Check sheet for the modelled part. Datum: model origin and axes. Units: mm. Face numbers are marked on the shaded views. A direction names the side the tool comes from. Round coordinates to 2 decimals unless told otherwise and drop trailing zeros. Order: outer loops, then holes, each group sorted by start corner. A loop starts at its lowest first (then second) coordinate and runs counter-clockwise, first axis right, second up. Notation, with made-up numbers: (67, 17) -> (115, 17) arc R13 ccw to (115, 38) -> close; hole circle Ø4 at (63.5, -8.75). An arc over 180 degrees is marked (long way). Answer in a Markdown table with one row per item. Add a question column.
1. Sectioned sample at D-D, the plane z = -20. Record the boundary of the cut face in (x, y), then the cut area to 3 significant figures.
2. Draft check along Z on the marked faces 1, 2, 3 and 4. Enter one of: +Z half, -Z half, draft (parallel to the pull), parting line (faces both ways), or undercut.
3. Material ranges on L1, parallel to Z at x = 0, y = 18; L2, parallel to X at y = -5.5, z = -19; L3, parallel to Y at x = -18.5, z = -28.5, recorded low to high. Write a range as from..to.
4. Sectioned sample at C-C, the plane y = 43. Record the boundary of the cut face in (x, z), then the cut area to 3 significant figures.
5. Sectioned sample at B-B, the plane z = -29. Record the boundary of the cut face in (x, y).
6. Sectioned sample at A-A, the plane x = 0. Record the boundary of the cut face in (y, z), then the cut area to 3 significant figures.
7. Access from +Z, -Z, +X, -X, +Y, -Y to the whole of each face (thin tool, end or side, straight path). Record for the marked faces 5, 6 and 7.
8. Depth check by flat-ended pin: P1, Ø4, axis at y = 41.5, z = 2.5, coming from the -X side; P2, Ø1, axis at y = 7.5, z = 3.5, coming from the -X side; P3, Ø1, axis at x = 11.5, y = 27.5, coming from the -Z side; P4, Ø8, axis at x = -8.5, z = -7, coming from the -Y side. Enter the tip coordinate at first touch or a pass-through.
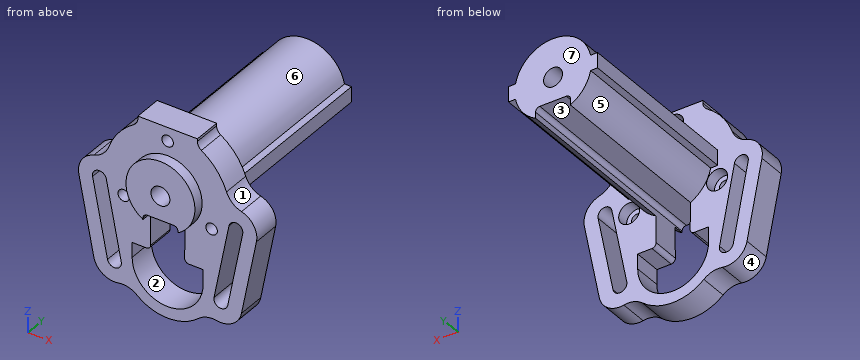
```python
from build123d import *

# Parameters (mm, degrees)
F1_DEPTH  = 8
F2_R      = 9.85
F3_DEPTH  = 3
F5_DEPTH  = 50
F6_R      = 2.7
F7_DEPTH  = 61
F8_R      = 3
F8_R_2    = 1.65
F9_DEPTH  = 3.3
F10_DEPTH = 25
F11_DEPTH = 25
F12_DEPTH = 25
F15_DEPTH = 61.001


with BuildPart() as f1:
    # F0 (on Front) → F1 (new body)
    with BuildSketch(Plane.XZ):
        with BuildLine():
            ThreePointArc((21.0969540743, 1.9835702793), (18.4718439184, 3.4572581024), (16.8204946757, 5.9744002934))
            ThreePointArc((16.8204946757, 5.9744002934), (13.9856503791, 11.0916222201), (9.6486486486, 15.0175257368))
            ThreePointArc((9.6486486486, 15.0175257368), (8.805873935, 15.9225674247), (8.5, 17.1208206579))
            Line((8.5, 17.1208206579), (8.5, 17.85))
            Line((8.5, 17.85), (0, 17.85))
            Line((0, 17.85), (-8.5, 17.85))
            Line((-8.5, 17.85), (-8.5, 17.1208206579))
            ThreePointArc((-8.5, 17.1208206579), (-8.805873935, 15.9225674247), (-9.6486486486, 15.0175257368))
            ThreePointArc((-9.6486486486, 15.0175257368), (-13.9856503791, 11.0916222201), (-16.8204946757, 5.9744002934))
            ThreePointArc((-16.8204946757, 5.9744002934), (-18.4718439184, 3.4572581024), (-21.0969540743, 1.9835702793))
            ThreePointArc((-21.0969540743, 1.9835702793), (-24.5891766283, -0.6435628298), (-25.3730516414, -4.9427472527))
            Line((-25.3730516414, -4.9427472527), (-21.10331181, -26.860989011))
            ThreePointArc((-21.10331181, -26.860989011), (-18.5752648191, -30.6838472237), (-14.0859973304, -31.6067469569))
            ThreePointArc((-14.0859973304, -31.6067469569), (-11.2665542119, -31.7051253732), (-8.7679800751, -33.0151120502))
            ThreePointArc((-8.7679800751, -33.0151120502), (0, -36.25), (8.7679800751, -33.0151120502))
            ThreePointArc((8.7679800751, -33.0151120502), (11.2665542119, -31.7051253732), (14.0859973304, -31.6067469569))
            ThreePointArc((14.0859973304, -31.6067469569), (18.5752648191, -30.6838472237), (21.10331181, -26.860989011))
            Line((21.10331181, -26.860989011), (25.3730516414, -4.9427472527))
            ThreePointArc((25.3730516414, -4.9427472527), (24.5891766283, -0.6435628298), (21.0969540743, 1.9835702793))
        make_face()
        with BuildLine():
            ThreePointArc((-21.4468540953, -4.1779120879), (-19.8661729047, -1.8323957325), (-17.5206565493, -3.4130769231))
            Line((-17.5206565493, -3.4130769231), (-13.2509167179, -25.3313186813))
            ThreePointArc((-13.2509167179, -25.3313186813), (-14.8315979085, -27.6768350368), (-17.177114264, -26.0961538462))
            Line((-17.177114264, -26.0961538462), (-21.4468540953, -4.1779120879))
        make_face(mode=Mode.SUBTRACT)
        with BuildLine():
            ThreePointArc((17.177114264, -26.0961538462), (14.8315979085, -27.6768350368), (13.2509167179, -25.3313186813))
            Line((13.2509167179, -25.3313186813), (17.5206565493, -3.4130769231))
            ThreePointArc((17.5206565493, -3.4130769231), (19.8661729047, -1.8323957325), (21.4468540953, -4.1779120879))
            Line((21.4468540953, -4.1779120879), (17.177114264, -26.0961538462))
        make_face(mode=Mode.SUBTRACT)
    extrude(amount=F1_DEPTH)

    # F2 (on face) → F3 (join)
    with BuildSketch(Plane.XZ.offset(8)):
        Circle(F2_R)
    extrude(amount=F3_DEPTH)

    # F4 (on face) → F5 (join)
    with BuildSketch(Plane(origin=(0, 0, 0), x_dir=(-1, 0, 0), z_dir=(0, 1, 0))):
        with BuildLine():
            Line((-12.73, -2.17), (-10.7328281455, -2.17))
            ThreePointArc((-10.7328281455, -2.17), (0, -10.95), (10.7328281455, -2.17))
            Line((10.7328281455, -2.17), (12.73, -2.17))
            Line((12.73, -2.17), (12.73, 2.17))
            Line((12.73, 2.17), (10.7328281455, 2.17))
            ThreePointArc((10.7328281455, 2.17), (0, 10.95), (-10.7328281455, 2.17))
            Line((-10.7328281455, 2.17), (-12.73, 2.17))
            Line((-12.73, 2.17), (-12.73, -2.17))
        make_face()
    extrude(amount=F5_DEPTH)

    # F6 (on face) → F7 (cut, through all)
    with BuildSketch(Plane.XZ.offset(11)):
        Circle(F6_R)
    extrude(amount=-F7_DEPTH, mode=Mode.SUBTRACT)

    # F8 (on face) → F9 (cut)
    with BuildSketch(Plane(origin=(0, 0, 0), x_dir=(-1, 0, 0), z_dir=(0, 1, 0))):
        with Locations((0, 14)):
            Circle(F8_R)
        with Locations((0, 14)):
            Circle(F8_R_2, mode=Mode.SUBTRACT)
        with Locations((-12.5570375793, -6.1903802172)):
            Circle(F8_R)
        with Locations((-12.5570375793, -6.1903802172)):
            Circle(F8_R_2, mode=Mode.SUBTRACT)
        with Locations((12.5570375793, -6.1903802172)):
            Circle(F8_R)
        with Locations((12.5570375793, -6.1903802172)):
            Circle(F8_R_2, mode=Mode.SUBTRACT)
    extrude(amount=-F9_DEPTH, mode=Mode.SUBTRACT)

    # F10 (cut): a face of the model
    f10_faces = [f1.faces().sort_by_distance(p)[0] for p in [
        (-12.5570375793, 0, -6.1903802172),
    ]]
    extrude(f10_faces, amount=-F10_DEPTH, mode=Mode.SUBTRACT)

    # F11 (cut): a face of the model
    f11_faces = [f1.faces().sort_by_distance(p)[0] for p in [
        (0, 0, 14),
    ]]
    extrude(f11_faces, amount=-F11_DEPTH, mode=Mode.SUBTRACT)

    # F12 (cut): a face of the model
    f12_faces = [f1.faces().sort_by_distance(p)[0] for p in [
        (12.5570375793, 0, -6.1903802172),
    ]]
    extrude(f12_faces, amount=-F12_DEPTH, mode=Mode.SUBTRACT)

    # F14 (on offset) → F15 (cut, through all)
    with BuildSketch(Plane.XZ.offset(-50)):
        with BuildLine():
            ThreePointArc((-4.8577252987, -17.4038723234), (-5.2034058164, -18.2628068545), (-6.057616918, -18.62))
            Line((-6.057616918, -18.62), (-10.14, -18.62))
            Line((-10.14, -18.62), (-10.14, -22.84))
            ThreePointArc((-10.14, -22.84), (0, -32.98), (10.14, -22.84))
            Line((10.14, -22.84), (10.14, -18.62))
            Line((10.14, -18.62), (6.057616918, -18.62))
            ThreePointArc((6.057616918, -18.62), (5.2034058164, -18.2628068545), (4.8577252987, -17.4038723234))
            Line((4.8577252987, -17.4038723234), (4.9836540955, -8.0348285577))
            ThreePointArc((4.9836540955, -8.0348285577), (4.6379735777, -7.1758940266), (3.7837624762, -6.8187008811))
            Line((3.7837624762, -6.8187008811), (0, -6.8187008811))
            Line((0, -6.8187008811), (-3.7837624762, -6.8187008811))
            ThreePointArc((-3.7837624762, -6.8187008811), (-4.6379735777, -7.1758940266), (-4.9836540955, -8.0348285577))
            Line((-4.9836540955, -8.0348285577), (-4.8577252987, -17.4038723234))
        make_face()
    extrude(amount=F15_DEPTH, mode=Mode.SUBTRACT)


solid = f1.part
```
Answer key:
| question | item | result |
|---|---|---|
| 1 | outline | (-22.44, -8) -> (-18.36, -8) -> (-18.36, 0) -> (-22.44, 0) -> close; (-14.29, -8) -> (-10.14, -8) -> (-10.14, 0) -> (-14.29, 0) -> close; (10.14, -8) -> (14.29, -8) -> (14.29, 0) -> (10.14, 0) -> close; (18.36, -8) -> (22.44, -8) -> (22.44, 0) -> (18.36, 0) -> close |
| 1 | area | 132 mm² |
| 2 | face 1 | +Z half |
| 2 | face 2 | undercut |
| 2 | face 3 | undercut |
| 2 | face 4 | -Z half |
| 3 | L1 | z = -6.82..-2.7, 2.7..10.95 |
| 3 | L2 | x = -22.63..-18.56, -14.48..-10.14, 10.14..14.48, 18.56..22.63 |
| 3 | L3 | y = -8..0 |
| 4 | outline | (-12.73, -2.17) -> (-10.73, -2.17) arc R10.95 ccw to (-4.96, -9.76) -> (-4.98, -8.03) arc R1.2 cw to (-3.78, -6.82) -> (3.78, -6.82) arc R1.2 cw to (4.98, -8.03) -> (4.96, -9.76) arc R10.95 ccw to (10.73, -2.17) -> (12.73, -2.17) -> (12.73, 2.17) -> (10.73, 2.17) arc R10.95 ccw to (-10.73, 2.17) -> (-12.73, 2.17) -> close; hole circle Ø5.4 at (0, 0) |
| 4 | area | 333 mm² |
| 5 | outline | (-20.23, -8) -> (-8.05, -8) -> (-8.05, 0) -> (-20.23, 0) -> close; (8.05, -8) -> (20.23, -8) -> (20.23, 0) -> (8.05, 0) -> close |
| 6 | outline | (-11, -6.82) -> (50, -6.82) -> (50, -2.7) -> (-11, -2.7) -> close; (-11, 2.7) -> (50, 2.7) -> (50, 10.95) -> (0, 10.95) -> (0, 11) -> (-3.3, 11) -> (-3.3, 12.35) -> (-8, 12.35) -> (-8, 9.85) -> (-11, 9.85) -> close; (-8, -36.25) -> (0, -36.25) -> (0, -32.98) -> (-8, -32.98) -> close; (-8, 15.65) -> (-3.3, 15.65) -> (-3.3, 17) -> (0, 17) -> (0, 17.85) -> (-8, 17.85) -> close |
| 6 | area | 797 mm² |
| 7 | face 5 | -Z, -X, +Y |
| 7 | face 6 | +Z, +Y |
| 7 | face 7 | +Z, -Z, +X, -X, +Y |
| 8 | P1 | stops at x = -12.73 |
| 8 | P2 | stops at x = -10.53 |
| 8 | P3 | stops at z = -2.17 |
| 8 | P4 | stops at y = -11 |
